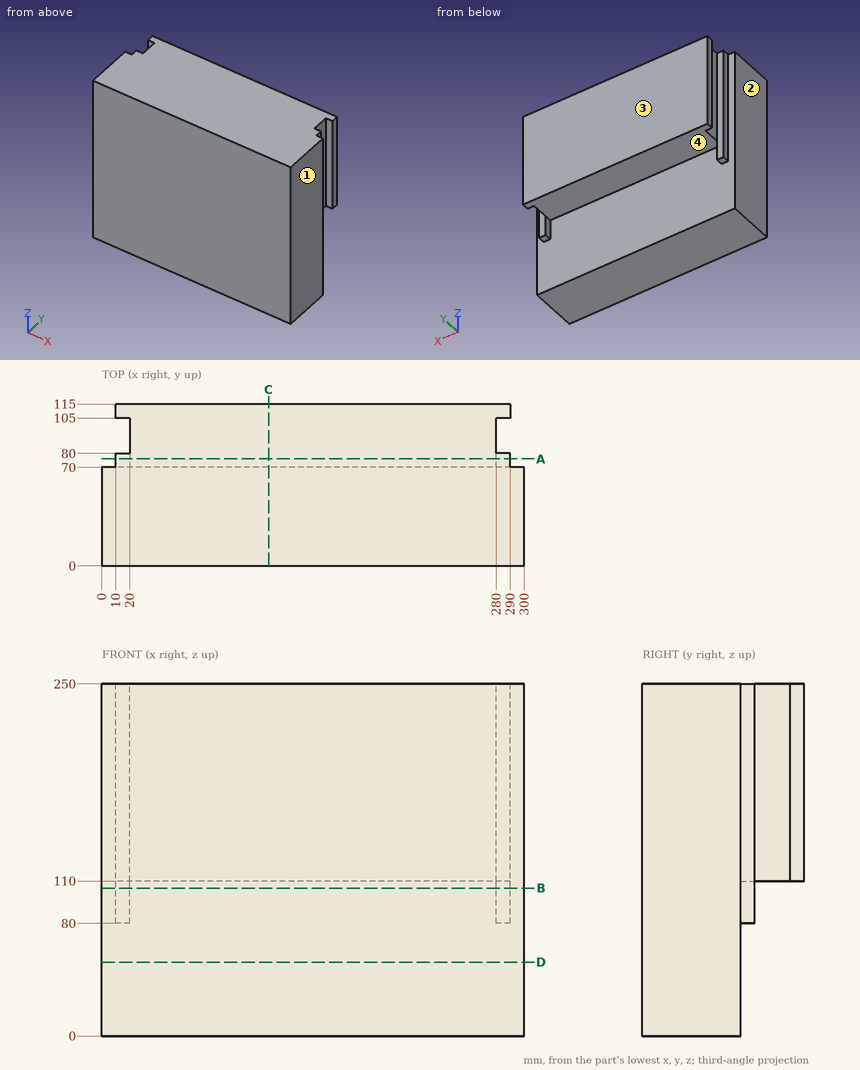
Check sheet for the drawn part. Datum: minimum x, y, z corner. Units: mm. Give positions to 0.01 mm unless a question says otherwise; leave off trailing zeros. Write each loop counter-clockwise with the first axis right and the second up, starting at its lowest first coordinate (ties: lowest second). Pieces come first, ordered by that corner, then holes. Notation, with made-up numbers: (48, -6) - (63, -6) arc R20 cw to (63, 33) - close; hole circle Ø3 at (10.5, 78). An arc over 180 degrees is marked (long way). Put each result on its own line as item: value.
1. Sectioned sample at D-D, the plane z = 52.5. Enter the section's corners in (x, y).
Ans:
outline: (0, 0) - (300, 0) - (300, 70) - (0, 70) - close
2. Sectioned sample at C-C, the plane x = 118.5. Enter the section's corners in (y, z), plus the area to 3 significant figures.
Ans:
outline: (0, 0) - (70, 0) - (70, 110) - (115, 110) - (115, 250) - (0, 250) - close
area: 23,800 mm²
3. Thickness scan on line 1 (Y direction, x = 285, z = 183); line 2 (Y direction, x = 229, z = 19.5); line 3 (Z direction, x = 65, y = 94). Record the ranges inside material, lowest first.
Ans:
line 1: y = 0 to 80, 105 to 115
line 2: y = 0 to 70
line 3: z = 110 to 250
4. Go/stop test with flat-tipped pins: pin 1 (12.5 mm diameter, centred on y = 95.5, z = 200, fed in from +X); pin 2 (5 mm diameter, centred on y = 112.5, z = 160, fed in from +X); pin 3 (3 mm diameter, centred on y = 73, z = 157, fed in from -X). Record where each tip stops, or that it passes through.
Ans:
pin 1: stops at x = 280
pin 2: stops at x = 290
pin 3: stops at x = 10
5. Sectioned sample at B-B, the plane z = 105. Enter the section's corners in (x, y).
Ans:
outline: (0, 0) - (300, 0) - (300, 70) - (290, 70) - (290, 80) - (280, 80) - (280, 70) - (20, 70) - (20, 80) - (10, 80) - (10, 70) - (0, 70) - close
6. Sectioned sample at A-A, the plane y = 76. Enter the section's corners in (x, z), plus the area to 3 significant figures.
Ans:
outline: (10, 80) - (20, 80) - (20, 110) - (280, 110) - (280, 80) - (290, 80) - (290, 250) - (10, 250) - close
area: 39,800 mm²
7. Draft check along X on the marked faces 1, 2, 3 and 4. Enter one of: +X half, -X half, draft (parallel to the pull), parting line (faces both ways), or undercut.
Ans:
face 1: +X half
face 2: -X half
face 3: draft
face 4: undercut
